Read the model definition and answer for the solid it produces. Units are mm, in the model's axes. Give positions to 0.01 mm unless a question says otherwise; leave off trailing zeros. Order: outer loops, then holes, each group sorted by start corner. A loop starts at its lowest first (then second) coordinate and runs counter-clockwise, first axis right, second up.
Item 1: A cutting plane is placed at B-B (y = 2863). Write down the section's boundary in (x, z).
Item 2: Find the intervals of material crossed by line 1 along Z through (x, y) = (-23093, 3140.5); line 2 along Z through (x, y) = (-22958, 3540.5); line 3 along Y through (x, z) = (-23085, 40095.5), in increasing order.
Item 3: A cutting plane is placed at A-A (x = -23301). Write down the section's boundary in (y, z).
Item 4: Given pin 1 Ø6 at (x, z) = (-23043.5, 40163) entering from -Y; pin 2 Ø2 at (x, z) = (-23019, 40224) entering from -Y; pin 3 Ø1.5 at (x, z) = (-23000, 40262.5) entering from +Y, each flat-ended and moving along its own axis, determine where each tip first touches the part or whether it passes through.
Item 5: A cutting plane is placed at D-D (z = 40503). Write down the section's boundary in (x, y).
Item 6: A cutting plane is placed at C-C (x = -23003). Write down the section's boundary in (y, z), plus the area to 3 significant figures.
from build123d import *

# Parameters (mm, degrees)
BOSS_EXTRUDE1_START = -22799.561142
BOSS_EXTRUDE1_DEPTH = 600
CUT_EXTRUDE1_START  = 2893.690104
CUT_EXTRUDE1_DEPTH  = 548.284271
BOSS_EXTRUDE2_DEPTH = 498
CUT_EXTRUDE2_DEPTH  = 694.125788176


with BuildPart() as part:
    # Sketch3 → Boss-Extrude1 (new body)
    with BuildSketch(Plane(origin=(0, 0, 0), x_dir=(0, 0, -1), z_dir=(1, 0, 0)).offset(BOSS_EXTRUDE1_START)):
        Polygon((-40199.900196056, 2810.990103756), (-41009.724036196, 3620.813943896), (-40995.581900573, 3634.95607952), (-40199.900196056, 2839.274375003), align=None)
    extrude(amount=-BOSS_EXTRUDE1_DEPTH)

    # Sketch4 → Cut-Extrude1 (cut)
    with BuildSketch(Plane(origin=(0, 0, 0), x_dir=(1, 0, 0), z_dir=(0, 1, 0)).offset(CUT_EXTRUDE1_START)):
        with BuildLine():
            Line((-22799.561141737, -40362.600196057), (-23030.561141738, -40362.600196057))
            ThreePointArc((-23030.561141738, -40362.600196057), (-23070.561141738, -40322.600196057), (-23030.561141738, -40282.600196057))
            Line((-23030.561141738, -40282.600196057), (-22799.561141737, -40282.600196057))
            Line((-22799.561141737, -40282.600196057), (-22799.561141737, -40362.600196057))
        make_face()
        with BuildLine():
            Line((-22799.561141737, -40802.600196057), (-22850.561141738, -40802.600196057))
            ThreePointArc((-22850.561141738, -40802.600196057), (-22890.561141738, -40762.600196057), (-22850.561141738, -40722.600196057))
            Line((-22850.561141738, -40722.600196057), (-22799.561141737, -40722.600196057))
            Line((-22799.561141737, -40722.600196057), (-22799.561141737, -40802.600196057))
        make_face()
    extrude(amount=CUT_EXTRUDE1_DEPTH, mode=Mode.SUBTRACT)

    # Sketch5 → Boss-Extrude2 (add)
    with BuildSketch(Plane.ZY.offset(23399.561141738)):
        Polygon((40057.780417375, 2668.870325074), (40199.900196056, 2810.990103756), (40199.900196056, 2839.274375003), (40043.638281751, 2683.012460698), align=None)
    extrude(amount=-BOSS_EXTRUDE2_DEPTH)

    # Sketch6 → Cut-Extrude2 (cut, through all)
    with BuildSketch(Plane(origin=(0, -18680.312910526, 18680.312910527), x_dir=(1, 0, 0), z_dir=(0, 0.707106781, -0.707106781))):
        with BuildLine():
            Line((-23349.561141737, -30397.304477375), (-23159.561141737, -30397.304477375))
            ThreePointArc((-23159.561141737, -30397.304477375), (-23149.561141737, -30387.304477375), (-23159.561141737, -30377.304477375))
            Line((-23159.561141737, -30377.304477375), (-23359.561141737, -30377.304477375))
            ThreePointArc((-23359.561141737, -30377.304477375), (-23366.632209549, -30380.233409563), (-23369.561141737, -30387.304477375))
            Line((-23369.561141737, -30387.304477375), (-23369.561141737, -31189.304477375))
            ThreePointArc((-23369.561141737, -31189.304477375), (-23366.632209549, -31196.375545187), (-23359.561141737, -31199.304477375))
            Line((-23359.561141737, -31199.304477375), (-22990.438858263, -31199.304477375))
            ThreePointArc((-22990.438858263, -31199.304477375), (-22980.438858263, -31189.304477375), (-22990.438858263, -31179.304477375))
            Line((-22990.438858263, -31179.304477375), (-23349.561141737, -31179.304477375))
            Line((-23349.561141737, -31179.304477375), (-23349.561141737, -31019.304477375))
            Line((-23349.561141737, -31019.304477375), (-22990.438858263, -31019.304477375))
            ThreePointArc((-22990.438858263, -31019.304477375), (-22980.438858263, -31009.304477375), (-22990.438858263, -30999.304477375))
            Line((-22990.438858263, -30999.304477375), (-23349.561141737, -30999.304477375))
            Line((-23349.561141737, -30999.304477375), (-23349.561141737, -30577.304477375))
            Line((-23349.561141737, -30577.304477375), (-23159.561141737, -30577.304477375))
            ThreePointArc((-23159.561141737, -30577.304477375), (-23149.561141737, -30567.304477375), (-23159.561141737, -30557.304477375))
            Line((-23159.561141737, -30557.304477375), (-23349.561141737, -30557.304477375))
            Line((-23349.561141737, -30557.304477375), (-23349.561141737, -30397.304477375))
        make_face()
    extrude(amount=-CUT_EXTRUDE2_DEPTH, mode=Mode.SUBTRACT)


solid = part.part
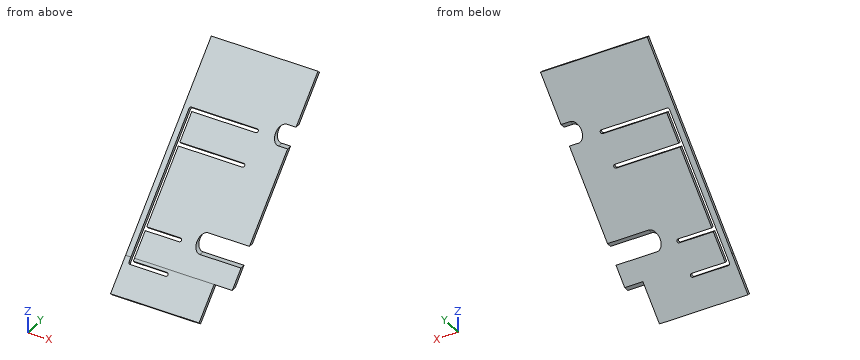
Response values:
1. outline: (-23399.56, 40223.63) - (-23369.56, 40223.63) - (-23369.56, 40251.91) - (-23399.56, 40251.91) - close; (-23349.56, 40223.63) - (-22799.56, 40223.63) - (-22799.56, 40251.91) - (-23349.56, 40251.91) - close
2. line 1: z = 40501.13 to 40529.41
2. line 2: z = 40901.13 to 40929.41
2. line 3: y = 2706.59 to 2734.87
3. outline: (2668.87, 40057.78) - (2683.01, 40043.64) - (2799.69, 40160.31) - (2785.54, 40174.45) - close; (2799.69, 40188.6) - (2813.83, 40174.45) - (2926.96, 40287.59) - (2912.82, 40301.73) - close; (2926.96, 40315.87) - (2941.11, 40301.73) - (3239.51, 40600.13) - (3225.36, 40614.27) - close; (3239.51, 40628.42) - (3253.65, 40614.27) - (3366.78, 40727.41) - (3352.64, 40741.55) - close; (3366.78, 40755.69) - (3380.93, 40741.55) - (3634.96, 40995.58) - (3620.81, 41009.72) - close
4. pin 1: stops at y = 2771.09
4. pin 2: stops at y = 2834.09
4. pin 3: stops at y = 2902.62
5. outline: (-23399.56, 3114.09) - (-23369.56, 3114.09) - (-23369.56, 3142.37) - (-23399.56, 3142.37) - close; (-23349.56, 3114.09) - (-22799.56, 3114.09) - (-22799.56, 3142.37) - (-23349.56, 3142.37) - close
6. outline: (2668.87, 40057.78) - (2683.01, 40043.64) - (2921.97, 40282.6) - (2893.69, 40282.6) - close; (2973.69, 40362.6) - (3001.97, 40362.6) - (3239.51, 40600.13) - (3225.36, 40614.27) - close; (3239.51, 40628.42) - (3253.65, 40614.27) - (3366.78, 40727.41) - (3352.64, 40741.55) - close; (3366.78, 40755.69) - (3380.93, 40741.55) - (3634.96, 40995.58) - (3620.81, 41009.72) - close
6. area: 23,900 mm2
